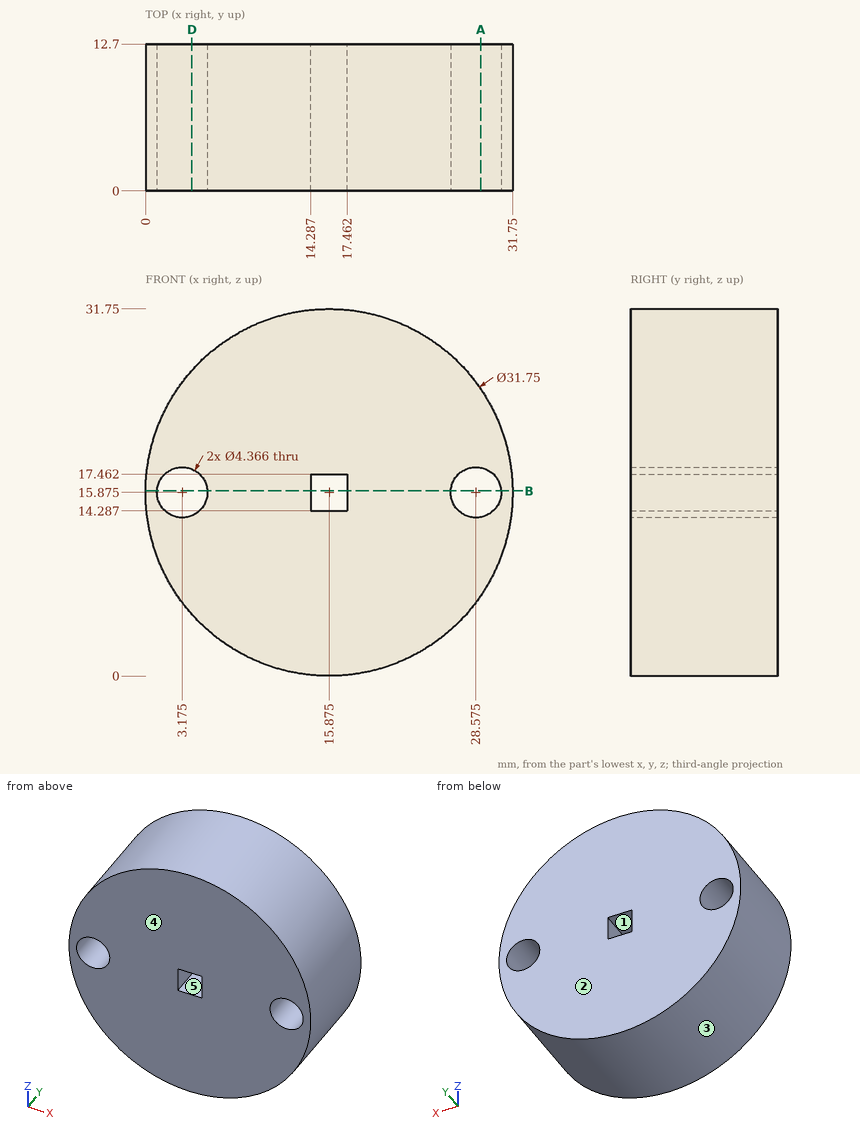
Input: dimensioned drawing with shaded views. Units: mm. Origin: part minimum x, y, z. A direction names the side the tool comes from. Give positions to 0.01 mm unless a question says otherwise; leave off trailing zeros. Write each loop counter-clockwise with the first axis right and the second up, starting at its lowest first coordinate (ties: lowest second). Pieces come first, ordered by that corner, then holes.
1. Pin query (flat end, axial travel): P1, Ø6, axis at x = 25, y = 7, coming from the +Z side; P2, Ø2, axis at y = 6.5, z = 13, coming from the -X side; P3, Ø6, axis at x = 4.5, y = 7, coming from the +Z side. Return the tip coordinate at first contact, or that it passes through.
2. Section query B-B, the plane z = 16. Count the separate pieces of the cut face and the enclosed holes in it, then the cut area to 3 significant figures.
3. Draft query along X for the marked faces 3, 4 and 5. Return one class per face: released by +X, released by -X, zero draft, split by the parting line, or undercut.
4. Reachability of the marked faces 1 and 2 from +Z, -Z, +X, -X, +Y, -Y: full face, straight path, thin tool, end or side. Return the list, or none.
5. Section query A-A, the plane x = 29. Return loops of the section in (y, z) (1 decimal).
6. Line query: probe 1 along X at (y, z) = (5.25, 15) (1 decimal); probe 2 along Z at (x, y) = (16.5, 12); probe 3 along Z at (x, y) = (10.5, 6.5). Output: solid intervals per line, ascending.
7. Section query D-D, the plane x = 4. Return loops of the section in (y, z) (1 decimal).
Computed:
1. P1: stops at z = 30.52
1. P2: stops at x = 0.11
1. P3: stops at z = 29.36
2. separate pieces: 4
2. enclosed holes: 0
2. area: 252 mm2
3. face 3: split by the parting line
3. face 4: zero draft
3. face 5: undercut
4. face 1: +Y, -Y
4. face 2: +Z, -Z, +X, -X, +Y
5. outline: (0, 6.9) - (12.7, 6.9) - (12.7, 13.7) - (0, 13.7) - close; (0, 18) - (12.7, 18) - (12.7, 24.8) - (0, 24.8) - close
6. probe 1: x = 0 to 1.2, 5.2 to 14.3, 17.5 to 26.6, 30.6 to 31.7
6. probe 2: z = 0.01 to 14.29, 17.46 to 31.74
6. probe 3: z = 0.94 to 30.81
7. outline: (0, 5.3) - (12.7, 5.3) - (12.7, 13.9) - (0, 13.9) - close; (0, 17.9) - (12.7, 17.9) - (12.7, 26.4) - (0, 26.4) - close
